```python
from build123d import *

# Parameters (mm, degrees)
F0_R     = 19.05
F1_DEPTH = 5.08
F2_T     = -1.27
F3_R     = 1.5875
F4_DEPTH = 3.175


with BuildPart() as f1:
    # F0 (on Front) → F1 (new body)
    with BuildSketch(Plane.XZ):
        Circle(F0_R)
    extrude(amount=F1_DEPTH)

    # F2
    f2_openings = [f1.faces().sort_by_distance(p)[0] for p in [
        (0, -5.08, 0),
    ]]
    offset(amount=F2_T, openings=f2_openings)

    # F3 (on face) → F4 (join)
    with BuildSketch(Plane.XZ.offset(1.27)):
        Circle(F3_R)
    extrude(amount=F4_DEPTH)


solid = f1.part
```
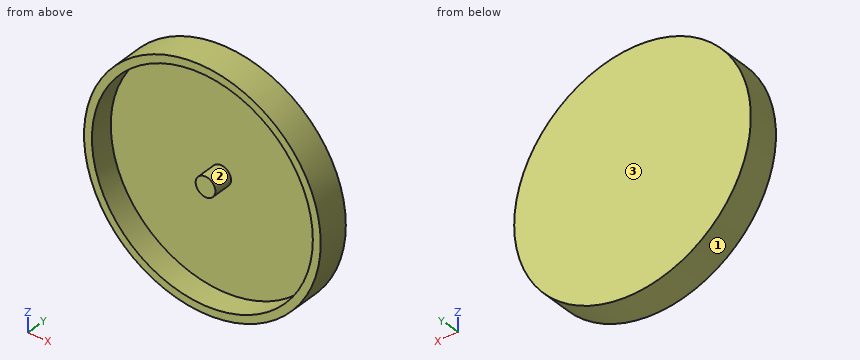
For this review, take the finished solid that the model builds, in its own axes (mm). Face numbers are marked on the shaded views. Coordinates: 2 decimals unless noted, no trailing zeros. Loops run counter-clockwise (first coordinate to the right, second up) from the corner with the lowest first, then second, coordinate; pieces in that order, holes last. Notation, with made-up numbers: (57, 71.5) -> (103, 71.5) arc R8 cw to (103, 85.5) -> close; hole circle Ø10 at (-13, -23.75). An arc over 180 degrees is marked (long way). Return JSON: item names as keys, results as strings. Group by question number.
(1) Consider section D-D, the plane y = -0.8. Give the boundary of the cut face in (x, z).
(2) Mouldability with a two-part tool opening along Z and no side actions: class the marked faces 1, 2 and 3 as pulls with the +Z half, pulls with the -Z half, needs draft (parallel to the pull), parting line crosses it, or undercut.
(3) For pin 1 Ø1.5 at (x, z) = (-4.5, -12) entering from +Y; pin 2 Ø1.5 at (x, y) = (3, -3.5) entering from -Z; pin 3 Ø10.5 at (x, z) = (2.5, 2.5) entering from -Y (3 decimals); pin 4 Ø2 at (x, y) = (11.5, -2.5) entering from +Z, all flat-tipped, find the tip position at first contact; note any pin that passes through.
(4) Consider section B-B, the plane y = -3. Count the separate pieces of the cut face and the enclosed holes in it, plus the area to 3 significant figures.
(5) To check wall thickness, follow L1, parallel to Z at x = 0, y = -3.1; L2, parallel to Y at x = -5, z = 9; L3, parallel to Z at x = -10, y = -3.55. State the ranges of each line that lie inside material, in increasing order.
Results below:
{
 "1": {"outline": "circle Ø38.1 at (0, 0)"},
 "2": {"face 1": "parting line crosses it", "face 2": "undercut", "face 3": "needs draft"},
 "3": {"pin 1": "stops at y = 0", "pin 2": "stops at z = -18.92", "pin 3": "stops at y = -4.445", "pin 4": "stops at z = 15.9"},
 "4": {"separate pieces": "2", "enclosed holes": "1", "area": "155 mm2"},
 "5": {"L1": "z = -19.05 to -17.78, -1.59 to 1.59, 17.78 to 19.05", "L2": "y = -1.27 to 0", "L3": "z = -16.21 to -14.7, 14.7 to 16.21"}
}
